The drawing under review shows one solid part. Ordinate dimensions are in mm from its lowest x, y, z. Coordinates: 2 decimals unless noted, no trailing zeros. Write each loop counter-clockwise with the first axis right and the second up, starting at its lowest first coordinate (ties: lowest second). Pieces come first, ordered by that corner, then holes.
Q1. Add section C-C, the plane z = 6.35. Give the boundary of the cut face in (x, y) (3 decimals).
Q2. To check wall thickness, follow probe 1 along X at (y, z) = (1.5, 2.5); probe 2 along X at (y, z) = (14.5, 6.35) (3 decimals); probe 3 along Z at (x, y) = (323.85, 16.75) (3 decimals). State the ranges of each line that lie inside material, in increasing order.
Q3. Add section A-A, the plane x = 57.15. Give the boundary of the cut face in (y, z) (3 decimals), plus the area to 3 significant figures.
Q4. Add section B-B, the plane y = 7. Give the boundary of the cut face in (x, z), plus the area to 3 significant figures.
Q5. Clearance check with flat-ended pins moving along their axes: pin 1 Ø6.5 at (x, z) = (323.5, 3.5) entering from -Y; pin 2 Ø5.5 at (x, z) = (323.85, 6.35) entering from -Y. State where each tip first meets the part, or that it passes through.
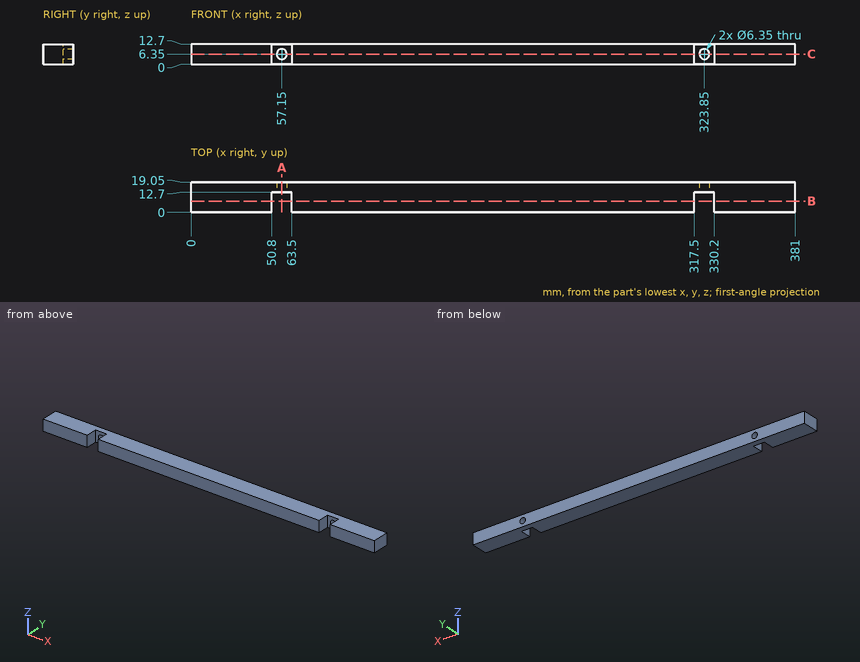
Here are the results:
1. outline: (0, 0) - (50.8, 0) - (50.8, 12.7) - (53.975, 12.7) - (53.975, 19.05) - (0, 19.05) - close; (60.325, 12.7) - (63.5, 12.7) - (63.5, 0) - (317.5, 0) - (317.5, 12.7) - (320.675, 12.7) - (320.675, 19.05) - (60.325, 19.05) - close; (327.025, 12.7) - (330.2, 12.7) - (330.2, 0) - (381, 0) - (381, 19.05) - (327.025, 19.05) - close
2. probe 1: x = 0 to 50.8, 63.5 to 317.5, 330.2 to 381
2. probe 2: x = 0 to 53.975, 60.325 to 320.675, 327.025 to 381
2. probe 3: z = 0 to 3.175, 9.525 to 12.7
3. outline: (12.7, 0) - (19.05, 0) - (19.05, 3.175) - (12.7, 3.175) - close; (12.7, 9.525) - (19.05, 9.525) - (19.05, 12.7) - (12.7, 12.7) - close
3. area: 40.3 mm2
4. outline: (0, 0) - (50.8, 0) - (50.8, 12.7) - (0, 12.7) - close; (63.5, 0) - (317.5, 0) - (317.5, 12.7) - (63.5, 12.7) - close; (330.2, 0) - (381, 0) - (381, 12.7) - (330.2, 12.7) - close
4. area: 4,520 mm2
5. pin 1: stops at y = 12.7
5. pin 2: passes through
